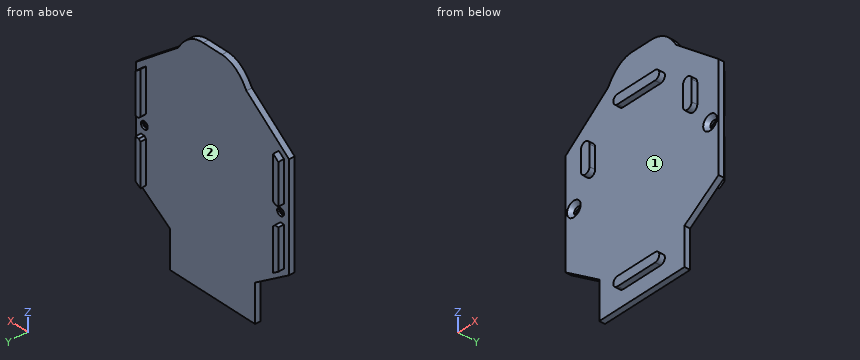
from build123d import *

# Parameters (mm, degrees)
BOSS_EXTRUDE1_DEPTH = 1.905
BOSS_EXTRUDE2_DEPTH = 3.81
SKETCH4_R           = 1.27
CUT_EXTRUDE1_DEPTH  = 3.81
CHAMFER1_SIZE       = 1.27
BOSS_EXTRUDE3_DEPTH = 1.905


with BuildPart() as part:
    # Sketch2 → Boss-Extrude1 (new body)
    with BuildSketch(Plane(origin=(0, 0, 0), x_dir=(1, 0, 0), z_dir=(0, 1, 0))):
        with BuildLine():
            Line((-28.22955712, 15.590722254), (-28.22955712, -19.997532082))
            Line((-28.22955712, -19.997532082), (-12.354557094, -32.697532128))
            add(Edge.make_bspline(
                [(-12.354557094, -32.697532128), (-10.357340532, -36.191853262), (-7.467085325, -39.002495951), (-3.133791164, -39.019277746)],
                knots=[0.450643599, 0.450643599, 0.450643599, 0.450643599, 1, 1, 1, 1], degree=3))
            Line((-3.133791164, -39.019277746), (3.824676923, -39.019277746))
            add(Edge.make_bspline(
                [(3.824676923, -39.019277746), (8.157971103, -39.002495951), (11.048226317, -36.191853237), (13.04544288, -32.697532082)],
                knots=[0.450643596, 0.450643596, 0.450643596, 0.450643596, 1, 1, 1, 1], degree=3))
            Line((13.04544288, -32.697532082), (28.92044288, -19.997532082))
            Line((28.92044288, -19.997532082), (28.92044288, 15.590722254))
            Line((28.92044288, 15.590722254), (16.22044288, 24.480722254))
            Line((16.22044288, 24.480722254), (16.22044288, 37.180722254))
            Line((16.22044288, 37.180722254), (-15.52955712, 37.180722254))
            Line((-15.52955712, 37.180722254), (-15.52955712, 24.480722254))
            Line((-15.52955712, 24.480722254), (-28.22955712, 15.590722254))
        make_face()
    extrude(amount=BOSS_EXTRUDE1_DEPTH)

    # Sketch3 → Boss-Extrude2 (add)
    with BuildSketch(Plane(origin=(0, 0, 0), x_dir=(1, 0, 0), z_dir=(0, 1, 0))):
        Polygon((-24.41955712, 1.606595086), (-24.41955712, 15.932373409), (-26.32455712, 14.598873409), (-26.32455712, 0.971595086), (-25.05455712, 0.971595086), align=None)
        Polygon((-24.41955712, -6.013404914), (-25.05455712, -5.378404914), (-26.32455712, -5.378404914), (-26.32455712, -19.081941748), (-24.41955712, -20.605941748), align=None)
        Polygon((27.01544288, 14.598873409), (25.11044288, 15.932373409), (25.11044288, 1.606595086), (25.74544288, 0.971595086), (27.01544288, 0.971595086), align=None)
        Polygon((27.01544288, -5.378404914), (25.74544288, -5.378404914), (25.11044288, -6.013404914), (25.11044288, -20.605941748), (27.01544288, -19.081941748), align=None)
    extrude(amount=BOSS_EXTRUDE2_DEPTH)

    # Sketch4 → Cut-Extrude1 (cut)
    with BuildSketch(Plane(origin=(0, 0, 0), x_dir=(1, 0, 0), z_dir=(0, 1, 0))):
        with Locations(Location((-25.05455712, -2.203404914, 0), (0, 0, 90))):
            Circle(SKETCH4_R)
        with Locations(Location((25.74544288, -2.203404914, 0), (0, 0, 90))):
            Circle(SKETCH4_R)
    extrude(amount=CUT_EXTRUDE1_DEPTH, mode=Mode.SUBTRACT)

    # Chamfer1
    chamfer1_edges = [part.edges().sort_by_distance(p)[0] for p in [
        (-25.05455712, 0, 3.473404914),
        (25.74544288, 0, 3.473404914),
    ]]
    chamfer(chamfer1_edges, length=CHAMFER1_SIZE)

    # Sketch5 → Boss-Extrude3 (add)
    with BuildSketch(Plane.XZ):
        with BuildLine():
            Line((-6.63955712, 26.9875), (7.33044288, 26.9875))
            ThreePointArc((7.33044288, 26.9875), (8.91794288, 25.4), (7.33044288, 23.8125))
            Line((7.33044288, 23.8125), (-6.63955712, 23.8125))
            ThreePointArc((-6.63955712, 23.8125), (-8.22705712, 25.4), (-6.63955712, 26.9875))
        make_face()
        with BuildLine():
            Line((-6.63955712, -28.8925), (7.33044288, -28.8925))
            ThreePointArc((7.33044288, -28.8925), (8.91794288, -30.48), (7.33044288, -32.0675))
            Line((7.33044288, -32.0675), (-6.63955712, -32.0675))
            ThreePointArc((-6.63955712, -32.0675), (-8.22705712, -30.48), (-6.63955712, -28.8925))
        make_face()
        with BuildLine():
            Line((-17.11705712, 17.111777746), (-17.11705712, 10.126777746))
            ThreePointArc((-17.11705712, 10.126777746), (-18.70455712, 8.539277746), (-20.29205712, 10.126777746))
            Line((-20.29205712, 10.126777746), (-20.29205712, 17.111777746))
            ThreePointArc((-20.29205712, 17.111777746), (-18.70455712, 18.699277746), (-17.11705712, 17.111777746))
        make_face()
        with BuildLine():
            Line((20.98294288, 17.111777746), (20.98294288, 10.126777746))
            ThreePointArc((20.98294288, 10.126777746), (19.39544288, 8.539277746), (17.80794288, 10.126777746))
            Line((17.80794288, 10.126777746), (17.80794288, 17.111777746))
            ThreePointArc((17.80794288, 17.111777746), (19.39544288, 18.699277746), (20.98294288, 17.111777746))
        make_face()
    extrude(amount=BOSS_EXTRUDE3_DEPTH)


solid = part.part
Check sheet for the modelled part. Datum: model origin and axes. Units: mm. Face numbers are marked on the shaded views. Round coordinates to 2 decimals unless told otherwise and drop trailing zeros. Loops run counter-clockwise (first coordinate to the right, second up) from the corner with the lowest first, then second, coordinate; pieces in that order, holes last. Notation, with made-up numbers: M 63.5,-24.5 L 83.5,-24.5 A31 cw 83.5,3.5 Z; hole C 80.5,-38.75 d11. An arc over 180 degrees is marked long. One line per question, with ' | ' between items. Start each with the question number.
Item 1: Section check D-D (z = -30.48). Record the boundary of the cut face in (x, y) (3 decimals).
Item 2: Section check A-A (y = -0.8). Record the boundary of the cut face in (x, z) (1 decimal), and give its area (3 significant figures).
Item 3: Section check B-B (z = 11). Record the boundary of the cut face in (x, y) (3 decimals).
Item 4: Scan lines: probe 1 along X at (y, z) = (-0.2, 12); probe 2 along Z at (x, y) = (1, -0.5); probe 3 along X at (y, z) = (3.4, 9.5). Record each from-to range of solid material in increasing order.
Item 5: Gauge pin test, flat ends, axial feed: pin 1 Ø0.6 at (y, z) = (3, 14.5) entering from -X; pin 2 Ø3 at (x, y) = (6, 2.5) entering from +Z; pin 3 Ø1 at (x, y) = (1.5, -1) entering from +Z. Record the tip position at first contact, or that the pin passes through.
Item 6: Section check C-C (z = 2.5). State how many separate pieces and enclosed holes the cut face has, and give its area (3 significant figures).
Item 7: Release check for a two-part mould opening along X. For the marked faces 1 and 2 record: released by +X, released by -X, zero draft, split by the parting line, or undercut.
Worked out:
1) outline: M -15.53,0 L -8.227,0 L -8.227,-1.905 L 8.918,-1.905 L 8.918,0 L 16.22,0 L 16.22,1.905 L -15.53,1.905 Z
2) outline: M -20.3,10.1 A1.6 ccw -17.1,10.1 L -17.1,17.1 A1.6 ccw -20.3,17.1 Z; M -6.6,-32.1 L 7.3,-32.1 A1.6 ccw 7.3,-28.9 L -6.6,-28.9 A1.6 ccw Z; M -6.6,23.8 L 7.3,23.8 A1.6 ccw 7.3,27 L -6.6,27 A1.6 ccw Z; M 17.8,10.1 A1.6 ccw 21,10.1 L 21,17.1 A1.6 ccw 17.8,17.1 Z | area: 165 mm^2
3) outline: M -28.23,0 L -20.292,0 L -20.292,-1.905 L -17.117,-1.905 L -17.117,0 L 17.808,0 L 17.808,-1.905 L 20.983,-1.905 L 20.983,0 L 28.92,0 L 28.92,1.905 L 27.015,1.905 L 27.015,3.81 L 25.11,3.81 L 25.11,1.905 L -24.42,1.905 L -24.42,3.81 L -26.325,3.81 L -26.325,1.905 L -28.23,1.905 Z
4) probe 1: -20.29 to -17.12, 17.81 to 20.98 | probe 2: -32.07 to -28.89, 23.81 to 26.99 | probe 3: -26.32 to -24.42, 25.11 to 27.02
5) pin 1: x = -26.32 | pin 2: z = 38.98 | pin 3: z = 26.99
6) separate pieces: 3 | enclosed holes: 0 | area: 96.2 mm^2
7) face 1: undercut | face 2: undercut
